The model under review builds one solid part; all positions refer to its coordinate system, in mm. A direction names the side the tool comes from. Coordinates: 2 decimals unless noted, no trailing zeros. Order: outer loops, then holes, each group sorted by start corner. A loop starts at its lowest first (then second) coordinate and runs counter-clockwise, first axis right, second up. Notation, with made-up numbers: (19, -19) - (31, -19) arc R26 ccw to (31, -1) - close; hole circle Ø9 at (33, 38). An arc over 180 degrees is marked (long way). Answer in a Markdown table with one row per item.
```python
from build123d import *

# Parameters (mm, degrees)
SKETCH1_W           = 91.6
SKETCH1_H           = 26.6
BOSS_EXTRUDE1_DEPTH = 6.3
SKETCH2_W           = 91.6
SKETCH2_H           = 53.8
BOSS_EXTRUDE2_DEPTH = 6
BOSS_EXTRUDE3_REACH = 108.941
SKETCH5_R           = 11.5
CUT_EXTRUDE1_DEPTH  = 56.5
SKETCH6_W           = 23
SKETCH6_H           = 11
CUT_EXTRUDE2_DEPTH  = 40
SKETCH8_R           = 1.6
CUT_EXTRUDE3_DEPTH  = 6
CUT_EXTRUDE4_REACH  = 111.225
SKETCH10_W          = 53.8
SKETCH10_H          = 10.6
CUT_EXTRUDE5_DEPTH  = 2.3
CUT_EXTRUDE6_REACH  = 97.014
SKETCH11_R          = 1.6


with BuildPart() as part:
    # Sketch1 → Boss-Extrude1 (new body)
    with BuildSketch(Plane(origin=(0, 0, 0), x_dir=(1, 0, 0), z_dir=(0, 1, 0))):
        with Locations((45.8, 13.3)):
            Rectangle(SKETCH1_W, SKETCH1_H)
    extrude(amount=BOSS_EXTRUDE1_DEPTH)

    # Sketch2 → Boss-Extrude2 (add)
    with BuildSketch(Plane(origin=(0, 6.3, 0), x_dir=(1, 0, 0), z_dir=(0, 1, 0))):
        with Locations((45.8, 13.3)):
            Rectangle(SKETCH2_W, SKETCH2_H)
    extrude(amount=BOSS_EXTRUDE2_DEPTH)

    # Boss-Extrude3: up to this face of the body (flat: up to its plane)
    boss_extrude3_end = Plane(part.part.faces().sort_by_distance((45.8, 9.3, -40.2))[0])
    # Sketch3 → Boss-Extrude3 (add, up to the picked face)
    with BuildSketch(Plane.XY.offset(13.6), mode=Mode.PRIVATE) as boss_extrude3_sk1:
        with BuildLine():
            Line((91.6, 12.3), (23.155649055, 17.195554695))
            ThreePointArc((23.155649055, 17.195554695), (17.419589145, 19.620522611), (15.1, 25.4))
            Line((15.1, 25.4), (-4, 25.4))
            Line((-4, 25.4), (0, 6.3))
            Line((0, 6.3), (0, 12.3))
            Line((0, 12.3), (91.6, 12.3))
        make_face()
    boss_extrude3_tool1 = split(extrude(boss_extrude3_sk1.sketch, amount=-BOSS_EXTRUDE3_REACH, mode=Mode.PRIVATE), bisect_by=boss_extrude3_end, keep=Keep.BOTH, mode=Mode.PRIVATE)
    add(boss_extrude3_tool1.solids().sort_by(Axis((22.17792, 16.713333, 13.6), (0, 0, -1)))[0])

    # Sketch5 → Cut-Extrude1 (cut, symmetric)
    with BuildSketch(Plane(origin=(1.263937397, 0.264698931, 0), x_dir=(0, 0, 1), z_dir=(-0.9787667222739368, -0.2049773240364267, 0))):
        with Locations((-13.3, 15)):
            Circle(SKETCH5_R)
    extrude(amount=CUT_EXTRUDE1_DEPTH, both=True, mode=Mode.SUBTRACT)

    # Sketch6 → Cut-Extrude2 (cut, symmetric)
    with BuildSketch(Plane(origin=(1.263937397, 0.264698931, 0), x_dir=(0, 0, 1), z_dir=(-0.9787667222739368, -0.2049773240364267, 0))):
        with Locations((-13.295563207, 20.180584042)):
            Rectangle(SKETCH6_W, SKETCH6_H)
    extrude(amount=CUT_EXTRUDE2_DEPTH, both=True, mode=Mode.SUBTRACT)

    # Sketch8 → Cut-Extrude3 (cut)
    with BuildSketch(Plane.XZ):
        with Locations(Location((15.8, -4.3, 0), (0, 0, 270))):
            Circle(SKETCH8_R)
        with Locations(Location((85.8, -4.3, 0), (0, 0, 270))):
            Circle(SKETCH8_R)
        with Locations(Location((85.8, -22.3, 0), (0, 0, 270))):
            Circle(SKETCH8_R)
        with Locations(Location((15.8, -22.3, 0), (0, 0, 270))):
            Circle(SKETCH8_R)
    extrude(amount=-CUT_EXTRUDE3_DEPTH, mode=Mode.SUBTRACT)

    # Cut-Extrude4: up to this face of the body (flat: up to its plane)
    cut_extrude4_end = Plane(part.part.faces().sort_by_distance((35.074761292, 12.665908848, -40.2))[0])
    # Sketch9 → Cut-Extrude4 (cut, up to the picked face)
    with BuildSketch(Plane.XY.offset(13.6), mode=Mode.PRIVATE) as cut_extrude4_sk1:
        with BuildLine():
            Line((-1.298429319, 12.5), (6.366705086, 12.5))
            Line((6.366705086, 12.5), (6.366705086, 23.1))
            Line((6.366705086, 23.1), (15.402527223, 23.1))
            ThreePointArc((15.402527223, 23.1), (15.168498155, 24.239113564), (15.1, 25.4))
            Line((15.1, 25.4), (-4, 25.4))
            Line((-4, 25.4), (-1.298429319, 12.5))
        make_face()
    cut_extrude4_tool1 = split(extrude(cut_extrude4_sk1.sketch, amount=-CUT_EXTRUDE4_REACH, mode=Mode.PRIVATE), bisect_by=cut_extrude4_end, keep=Keep.BOTH, mode=Mode.PRIVATE)
    add(cut_extrude4_tool1.solids().sort_by(Axis((3.156249, 20.011038, 13.6), (0, 0, -1)))[0], mode=Mode.SUBTRACT)

    # Sketch10 → Cut-Extrude5 (cut)
    with BuildSketch(Plane.ZY.offset(-6.366705086)):
        with Locations((-13.3, 17.8)):
            Rectangle(SKETCH10_W, SKETCH10_H)
    extrude(amount=-CUT_EXTRUDE5_DEPTH, mode=Mode.SUBTRACT)

    # Sketch11 → Cut-Extrude6 (cut, up to next)
    with BuildSketch(Plane.ZY.offset(-8.666705086), mode=Mode.PRIVATE) as cut_extrude6_sk1:
        with Locations((-35.3, 17.65)):
            Circle(SKETCH11_R)
    cut_extrude6_tool1 = extrude(cut_extrude6_sk1.sketch, amount=-CUT_EXTRUDE6_REACH, mode=Mode.PRIVATE) & part.part
    # Sketch11 → Cut-Extrude6 (cut, up to next)
    with BuildSketch(Plane.ZY.offset(-8.666705086), mode=Mode.PRIVATE) as cut_extrude6_sk2:
        with Locations((8.7, 17.65)):
            Circle(SKETCH11_R)
    cut_extrude6_tool2 = extrude(cut_extrude6_sk2.sketch, amount=-CUT_EXTRUDE6_REACH, mode=Mode.PRIVATE) & part.part
    add(cut_extrude6_tool1.solids().sort_by_distance((8.666705, 17.65, -35.3))[0], mode=Mode.SUBTRACT)
    add(cut_extrude6_tool2.solids().sort_by_distance((8.666705, 17.65, 8.7))[0], mode=Mode.SUBTRACT)


solid = part.part
```
Item 1: Tool access review of faces 4 (the face through (8.667, 18, 5)), 5 (the face through (45, 3, 0)), 6 (the face through (87.386, 2.958, -22.092)): name each direction out of +Z, -Z, +X, -X, +Y, -Y from which nothing blocks a thin tool from reaching the whole face with its end or side.
Check values:
| item | result |
|---|---|
| face 4 | +Z, -Z, -X, +Y |
| face 5 | +Z, +X, -X, -Y |
| face 6 | -Y |
Item 2: Clearance check with flat-ended pins moving along their axes: pin 1 Ø3.5 at (x, z) = (86.5, -22.5) entering from -Y; pin 2 Ø1 at (x, y) = (36, 5.5) entering from +Z; pin 3 Ø3 at (x, z) = (64, -30.5) entering from +Y; pin 4 Ø8 at (x, z) = (3.5, 3.5) entering from +Y. State where each tip first meets the part, or that it passes through.
Check values:
| item | result |
|---|---|
| pin 1 | y = 0 |
| pin 2 | z = 0 |
| pin 3 | y = 14.38 |
| pin 4 | y = 12.5 |
Item 3: We need section B-B, the plane y = 20.25. Write out the cut boundary in (x, z), then the cut area to 3 significant figures.
Check values:
| item | result |
|---|---|
| outline | (8.67, -40.2) - (16.86, -40.2) - (16.86, -24.8) - (8.67, -24.8) - close; (8.67, -1.8) - (16.86, -1.8) - (16.86, 13.6) - (8.67, 13.6) - close |
| area | 252 mm^2 |
Item 4: Mouldability with a two-part tool opening along X and no side actions: class faces 1 (the face through (0, 2, -13)), 2 (the face through (16, 6, -4)), 3 (the face through (45, 11, 13.6)) as +X half, -X half, draft (parallel to the pull), parting line (faces both ways), or undercut.
Check values:
| item | result |
|---|---|
| face 1 | -X half |
| face 2 | undercut |
| face 3 | draft |
Item 5: We need section C-C, the plane z = 8.7. Write out the cut boundary in (x, y), then the cut area to 3 significant figures.
Check values:
| item | result |
|---|---|
| outline | (-1.3, 12.5) - (0, 6.3) - (91.6, 6.3) - (91.6, 12.3) - (39.17, 16.05) - (8.67, 16.05) - (8.67, 12.5) - close; (8.67, 19.25) - (17.81, 19.25) arc R8.1 cw to (15.4, 23.1) - (8.67, 23.1) - close |
| area | 798 mm^2 |
Item 6: To check wall thickness, follow line 1 (Z direction, x = 85.8, y = 1.8); line 2 (X direction, y = 2.2, z = -22.3); line 3 (Z direction, x = 25.5, y = 16.25). State the ranges of each line that lie inside material, in increasing order. Write a range as from..to.
Check values:
| item | result |
|---|---|
| line 1 | -26.6..-23.9, -20.7..-5.9, -2.7..0 |
| line 2 | 0..14.2, 17.4..84.2, 87.4..91.6 |
| line 3 | -40.2..-36.07, -34.53..-23.96, -2.64..7.93, 9.47..13.6 |
Item 7: We need section D-D, the plane x = 66. Write out the cut boundary in (y, z).
Check values:
| item | result |
|---|---|
| outline | (0, -26.6) - (6.3, -26.6) - (6.3, -40.2) - (14.13, -40.2) - (14.13, 13.6) - (6.3, 13.6) - (6.3, 0) - (0, 0) - close |
Item 8: We need section A-A, the plane z = 2. Write out the cut boundary in (x, y).
Check values:
| item | result |
|---|---|
| outline | (-1.3, 12.5) - (0, 6.3) - (91.6, 6.3) - (91.6, 12.3) - (23.16, 17.2) arc R8.1 cw to (15.4, 23.1) - (8.67, 23.1) - (8.67, 12.5) - close |
